The listing builds one solid part. Answer for the finished solid, in the listing's coordinates (mm). A direction names the side the tool comes from. Coordinates: 2 decimals unless noted, no trailing zeros. Loops run counter-clockwise (first coordinate to the right, second up) from the corner with the lowest first, then second, coordinate; pieces in that order, holes last. Notation, with made-up numbers: (-15, -23) - (-3, -23) arc R25 ccw to (-3, 2) - close; hole circle Ø3 at (28.5, 0.25). An arc over 180 degrees is marked (long way). Write each question's results on one line, items separated by ' | '. Start each with the question number.
(1) Find section A-A on y = 25.5. Determine the outline of the cut face in (x, z).
(2) Determine the mould class of faces 6 (the flat face through (0, 32.5, -2)), 7 (the flat face through (-10, 23.5, 0)), 8 (the flat face through (0, 39, -0.96)) for opening direction Z: released by +Z, released by -Z, zero draft, split by the parting line, or undercut.
(3) For faces 1 (the flat face through (7, 27, -0.5)), 2 (the flat face through (-5, -0.5, 11.1)), 3 (the flat face through (3, 30.5, 0)), 4 (the flat face through (-8.8, 28.5, 0)), 5 (the flat face through (-7, 27, 0.5)), determine the directions among +Z, -Z, +X, -X, +Y, -Y from which every point of the face is accessible in a straight line to the end or side of a thin tool.
(4) Find section C-C on x = 0. Determine the outline of the cut face in (y, z), then the cut area to 3 significant figures.
(5) Consider line 1 (X direction, y = 24.6, z = 0); line 2 (Z direction, x = 10.04, y = 26.8); line 3 (Y direction, x = 6, z = -8.75). Determine where each line is inside the solid, lowest interval first. Write a range as from..to.
(6) Find section D-D on y = -6. Determine the outline of the cut face in (x, z).
(7) Find section B-B on z = -8. Determine the outline of the cut face in (x, y).
(8) Given pin 1 Ø8 at (x, y) = (-11, -14) entering from +Z; pin 2 Ø1.4 at (x, y) = (-1, 36) entering from -Z; pin 3 Ø1.5 at (x, y) = (7, 27) entering from -Z; pin 4 Ø8 at (x, y) = (3, 10) entering from -Z, each flat-ended and moving along its own axis, determine where each tip first touches the part or whether it passes through.
from build123d import *

# Parameters (mm, degrees)
CROQUIS1_W              = 2.5
CROQUIS1_H              = 14
CORTAR_EXTRUIR1_DEPTH   = 12
CROQUIS4_R              = 2.25
CROQUIS4_R_2            = 0.9
CROQUIS4_W              = 18
CROQUIS4_H              = 1
SALIENTE_EXTRUIR1_DEPTH = 5


with BuildPart() as part:
    # Croquis1 → Revolución1 (revolve)
    with BuildSketch(Plane.XY):
        with Locations((-1.25, 37.5)):
            Rectangle(CROQUIS1_W, CROQUIS1_H)
        Polygon((-12, -30.5), (0, -30.5), (0, 30.5), (-6.5, 30.5), (-6.5, 26.5), (-9.15, 26.5), (-9.15, 23.5), (-13.65, 23.5), (-13.65, -0.5), (-12, -0.5), align=None)
    revolve(axis=Axis((0, 65.687156563, 0), (0, -1, 0)))

    # Croquis2 → Cortar-Extruir1 (cut)
    with BuildSketch(Plane(origin=(0, 44.5, 0), x_dir=(1, 0, 0), z_dir=(0, 1, 0))):
        Polygon((-55.580517034, 0.96), (-2.308332732, 0.96), (2.308332732, 0.96), (55.580517034, 0.96), (55.580517034, 107.504368605), (-55.580517034, 107.504368605), align=None)
    extrude(amount=-CORTAR_EXTRUIR1_DEPTH, mode=Mode.SUBTRACT)

    # Croquis4 → Saliente-Extruir1 (add)
    with BuildSketch(Plane(origin=(0, 23.5, 0), x_dir=(1, 0, 0), z_dir=(0, 1, 0))):
        with Locations((-10.04, 0)):
            Circle(CROQUIS4_R)
        with Locations((-10.04, 0)):
            Circle(CROQUIS4_R_2, mode=Mode.SUBTRACT)
        with Locations((10.04, 0)):
            Circle(CROQUIS4_R)
        with Locations((10.04, 0)):
            Circle(CROQUIS4_R_2, mode=Mode.SUBTRACT)
        Rectangle(CROQUIS4_W, CROQUIS4_H)
    extrude(amount=SALIENTE_EXTRUIR1_DEPTH)


solid = part.part
Values:
1) outline: (-8.94, -1.96) arc R9.15 ccw to (8.94, -1.96) arc R2.25 ccw (long way) to (8.94, 1.96) arc R9.15 ccw to (-8.94, 1.96) arc R2.25 ccw (long way) to start; hole (-9.15, -0.13) arc R9.15 cw to (-9.15, 0.13) arc R0.9 ccw (long way) to start; hole (9.15, -0.13) arc R0.9 ccw (long way) to (9.15, 0.13) arc R9.15 cw to start
2) face 6: zero draft | face 7: undercut | face 8: released by -Z
3) face 1: -Z, +Y | face 2: -Y | face 3: +Y | face 4: +Z, -Z, -X, +Y | face 5: +Z, +Y
4) outline: (-30.5, -12) - (-0.5, -12) - (-0.5, -13.65) - (23.5, -13.65) - (23.5, -9.15) - (26.5, -9.15) - (26.5, -6.5) - (30.5, -6.5) - (30.5, -2.5) - (32.5, -2.5) - (32.5, -0.96) - (44.5, -0.96) - (44.5, 2.5) - (30.5, 2.5) - (30.5, 6.5) - (26.5, 6.5) - (26.5, 9.15) - (23.5, 9.15) - (23.5, 13.65) - (-0.5, 13.65) - (-0.5, 12) - (-30.5, 12) - close | area: 1,530 mm²
5) line 1: x = -12.29..-10.94, -9.15..9.15, 10.94..12.29 | line 2: z = -2.25..-0.9, 0.9..2.25 | line 3: y = -30.5..23.5
6) outline: circle Ø24 at (0, 0)
7) outline: (-11.06, -0.5) - (-8.94, -0.5) - (-8.94, -30.5) - (8.94, -30.5) - (8.94, -0.5) - (11.06, -0.5) - (11.06, 23.5) - (4.44, 23.5) - (4.44, 26.5) - (-4.44, 26.5) - (-4.44, 23.5) - (-11.06, 23.5) - close
8) pin 1: stops at z = 9.75 | pin 2: stops at z = -0.96 | pin 3: stops at z = -6.5 | pin 4: stops at z = -13.65
